Read the model definition and answer for the solid it produces. Units are mm, in the model's axes. A direction names the side the tool comes from. Coordinates: 2 decimals unless noted, no trailing zeros. Order: outer loops, then holes, each group sorted by start corner. A loop starts at its lowest first (then second) coordinate and runs counter-clockwise, first axis right, second up. Notation, with made-up numbers: M 28,62 L 48,62 A24 ccw 48,101 Z; hole C 39.25,-34.75 d10. An arc over 180 degrees is marked long. One line per question, with ' | ' between items. Start each with the question number.
1) Consider probe 1 along Z at (x, y) = (18.5, 2.2); probe 2 along Z at (x, y) = (19, 2.75); probe 3 along Z at (x, y) = (-43.5, 1.5). Determine where each line is inside the solid, lowest interval first.
2) A tool of negligible diameter and unlimited length cuts with its end or side. For faces 5 (the face through (26.69, 1.61, -36.27)), 6 (the face through (1, 0, -1)), 7 (the face through (-45, 2, -4.978)), 8 (the face through (18.15, 1.61, -41.39)), 9 (the face through (26.77, 1.61, 36.41)), from which of +Z, -Z, +X, -X, +Y, -Y can it reach the whole face along a straight path? Write none if from no direction.
3) Find section B-B, the plane x = -31. Write down the section's boundary in (y, z) (3 decimals).
4) The mould has two halves that part along X. Classify faces 1 (the face through (50.796, 1.565, 0.675)), 2 (the face through (-39.125, 2, 0)), 3 (the face through (19.62, 1.61, -33.85)), 4 (the face through (-25.982, 1.565, 43.653)): +X half, -X half, draft (parallel to the pull), parting line (faces both ways), or undercut.
5) Find section A-A, the plane y = 2.2. Write down the section's boundary in (x, z).
6) Given P1, Ø1.6, axis at x = -44, y = 2, coming from the +Z side; P2, Ø1.5, axis at x = 10.5, y = 2, coming from the +Z side; P3, Ø1.6, axis at x = -45, y = 2, coming from the -Z side, each flat-ended and moving along its own axis, determine where each tip first touches the part or whether it passes through.
7) Find section C-C, the plane z = -30. Write down the section's boundary in (x, y) (3 decimals), plus the area to 3 significant figures.
from build123d import *

# Parameters (mm, degrees)
SKETCH1_R         = 50.8
EXTRUDE1_DEPTH    = 3.175
EXTRUDE2_DEPTH    = 72.912172996
CIRPATTERN1_COUNT = 2
CIRPATTERN1_ANGLE = 120
CIRPATTERN2_COUNT = 2
CIRPATTERN2_ANGLE = 120


with BuildPart() as part:
    # Sketch1 → Extrude1 (new body)
    with BuildSketch(Plane(origin=(0, 0, 0), x_dir=(1, 0, 0), z_dir=(0, 1, 0))):
        with Locations(Location((0, 0, 0), (0, 0, 270))):
            Circle(SKETCH1_R)
    extrude(amount=EXTRUDE1_DEPTH)

    # Sketch3 → Extrude2 (cut, through all)
    with BuildSketch(Plane(origin=(0, 3.175, 0), x_dir=(-1, 0, 0), z_dir=(0, 1, 0))):
        Polygon((42.177913697, -4.9784), (39.125469867, -4.9784), (39.125469867, 4.9784), (42.300469867, 4.9784), (50.555469867, 4.9784), (52.750339101, 4.9784), (52.750339101, -4.9784), (50.555469867, -4.9784), align=None)
    extrude2 = extrude(amount=-EXTRUDE2_DEPTH, mode=Mode.SUBTRACT)

    # CirPattern1: Extrude2 ×2 about axis
    cirpattern1_axis = Axis((0, 38.178274824, 0), (0, -1, 0))
    for i in range(1, CIRPATTERN1_COUNT):
        add(extrude2.rotate(cirpattern1_axis, i * CIRPATTERN1_ANGLE / (CIRPATTERN1_COUNT - 1)), mode=Mode.SUBTRACT)

    # CirPattern2: Extrude2 ×2 about axis
    cirpattern2_axis = Axis((0, 0, 0), (0, 1, 0))
    for i in range(1, CIRPATTERN2_COUNT):
        add(extrude2.rotate(cirpattern2_axis, i * CIRPATTERN2_ANGLE / (CIRPATTERN2_COUNT - 1)), mode=Mode.SUBTRACT)


solid = part.part
Report:
1) probe 1: z = -47.31 to -42, -34.5 to 34.5, 42 to 47.31 | probe 2: z = -47.11 to -42.87, -34.21 to 34.21, 42.87 to 47.11 | probe 3: z = -26.24 to -4.98, 4.98 to 26.24
2) face 5: -Z, +Y, -Y | face 6: +Z, -Z, +X, -X, -Y | face 7: -X, +Y, -Y | face 8: +Y, -Y | face 9: +Z, +Y, -Y
3) outline: M 0,-40.245 L 3.175,-40.245 L 3.175,40.245 L 0,40.245 Z
4) face 1: +X half | face 2: -X half | face 3: undercut | face 4: parting line
5) outline: M -50.56,-4.98 A50.8 ccw 20.97,-46.27 L 15.25,-36.37 L 23.87,-31.39 L 29.59,-41.29 A50.8 ccw 29.59,41.29 L 23.87,31.39 L 15.25,36.37 L 20.97,46.27 A50.8 ccw -50.56,4.98 L -39.13,4.98 L -39.13,-4.98 Z
6) P1: stops at z = 26.73 | P2: stops at z = 49.86 | P3: stops at z = -25.04
7) outline: M -40.996,0 L 40.996,0 L 40.996,3.175 L -40.996,3.175 Z | area: 260 mm^2
